Autodesk Inventor part; units mm, degrees
ref_plane "YZ Plane" through (0, 0, 0) normal (1, 0, 0) x (0, 1, 0)
ref_plane "XZ Plane" through (0, 0, 0) normal (0, 1, 0) x (-1, 0, 0)
ref_plane "XY Plane" through (0, 0, 0) normal (0, 0, 1) x (1, 0, 0)
sketch "Sketch1" plane through (0, 0, 0) normal (0, 1, 0) x (-1, 0, 0)
  line L0 (-24.384, 42.545) -> (24.384, 42.545)
  line L1 (24.384, 42.545) -> (24.384, -42.545)
  line L2 (24.384, -42.545) -> (-24.384, -42.545)
  line L3 (-24.384, -42.545) -> (-24.384, 42.545)
  line L4 (-24.384, 42.545) -> (24.384, -42.545) construction
  line L5 (24.384, 42.545) -> (-24.384, -42.545) construction
  line L6 (-12.7, 36.83) -> (12.7, 36.83)
  line L7 (12.7, 36.83) -> (12.7, -36.83)
  line L8 (12.7, -36.83) -> (-12.7, -36.83)
  line L9 (-12.7, -36.83) -> (-12.7, 36.83)
  line L10 (-12.7, 36.83) -> (12.7, -36.83) construction
  line L11 (12.7, 36.83) -> (-12.7, -36.83) construction
  line L12 (-24.384, 42.545) -> (-34.925, 42.545)
  line L13 (-34.925, 42.545) -> (-34.925, -42.545)
  line L14 (-34.925, -42.545) -> (-24.384, -42.545)
  line L15 (-24.384, -42.545) -> (-24.384, 42.545)
  circle A0 centre (15.494, 37.465) radius 1.5875
  circle A1 centre (-15.494, 37.465) radius 1.5875
  circle A2 centre (-15.494, -37.465) radius 1.5875
  circle A3 centre (15.494, -37.465) radius 1.5875
  point P0 (0, 0)
  dimension "d0" = 73.66
  dimension "d1" = 25.4
  dimension "d4" = 85.09
  dimension "d5" = 34.925
  dimension "d6" = 59.309
  dimension "d7" = 3.175
  dimension "d8" = 3.175
  dimension "d9" = 3.175
  dimension "d10" = 3.175
  dimension "d11" = 5.08
  dimension "d12" = 8.89
  dimension "d13" = 5.08
  dimension "d14" = 19.431
extrude "Extrusion1" add sketch "Sketch1" along normal blind 6.985
sketch "Sketch3" plane through (0, 0, 0) normal (0, -1, 0) x (1, 0, 0)
  line L0 (34.925, 42.545) -> (34.925, -42.545)
  line L1 (34.925, -42.545) -> (17.78, -42.545)
  line L2 (17.78, -42.545) -> (17.78, -5.715)
  line L3 (17.78, -5.715) -> (34.925, -5.715)
  line L4 (34.925, -5.715) -> (34.925, -42.545)
  point P0 (0, 0)
  point P1 (34.925, -5.715)
  dimension "d31" = 36.83
  dimension "d32" = 17.145
extrude "Extrusion3" add sketch "Sketch3" along normal blind 8.89
sketch "Sketch2" plane through (0, 6.985, 0) normal (0, 1, 0) x (1, 0, 0)
  circle A0 centre (21.59, 29.21) radius 3.0162
  circle A1 centre (28.194, 29.21) radius 3.0162
  circle A2 centre (24.638, 38.1) radius 3.0162
  circle A3 centre (24.638, 19.812) radius 3.0162
  line L0 (34.925, -42.545) -> (34.925, 42.545)
  circle A4 centre (24.638, 9.8298) radius 3.0162
  line L1 (34.925, 42.545) -> (-24.384, 42.545)
  point P0 (0, 0)
  dimension "d17" = 6.0325
  dimension "d18" = 6.0325
  dimension "d19" = 6.0325
  dimension "d20" = 6.0325
  dimension "d21" = 6.731
  dimension "d22" = 10.287
  dimension "d23" = 13.335
  dimension "d24" = 6.0325
  dimension "d25" = 4.445
  dimension "d26" = 18.288
  dimension "d27" = 8.89
  dimension "d28" = 28.2702
extrude "Extrusion2" cut sketch "Sketch2" against normal through all
sketch "Sketch7" plane through (-24.384, 0, -42.545) normal (0, 0, -1) x (-1, 0, 0)
  line L0 (-59.309, 6.985) -> (0, 6.985)
  line L1 (0, 0) -> (-59.309, 0)
  line L2 (0, 6.985) -> (-59.309, 6.985)
  line L3 (-59.309, 6.985) -> (-59.309, 0)
  line L4 (-59.309, 0) -> (0, 0)
  line L5 (0, 0) -> (0, 6.985)
  line L6 (-42.164, -8.89) -> (-59.309, -8.89)
  line L7 (-59.309, -8.89) -> (-42.164, -8.89)
  line L8 (-42.164, -8.89) -> (-42.164, 0)
  line L9 (-42.164, 0) -> (-59.309, 0)
  line L10 (-59.309, 0) -> (-59.309, -8.89)
  point P0 (-24.384, 0)
  point P1 (-45.4299, 3.81)
  point P2 (-45.4299, 3.81)
extrude "Extrusion5" add sketch "Sketch7" along normal blind 2.54
sketch "Sketch4" plane through (0, 6.985, 0) normal (0, 1, 0) x (1, 0, 0)
  circle A0 centre (21.59, 29.21) radius 3.0162
  circle A1 centre (21.59, 29.21) radius 5.715
  circle A2 centre (24.638, 38.1) radius 3.0162
  circle A3 centre (24.638, 38.1) radius 5.715
  circle A4 centre (28.194, 29.21) radius 3.0162
  circle A5 centre (24.638, 19.812) radius 3.0162
  circle A6 centre (24.638, 19.812) radius 5.715
  circle A7 centre (24.638, 9.8298) radius 3.0162
  circle A8 centre (24.638, 9.8298) radius 5.715
  circle A9 centre (28.194, 29.21) radius 5.715
  point P0 (0, 0)
  point P1 (24.892, 24.5455)
  point P2 (24.892, 33.8745)
  point P3 (23.8684, 25.4749)
  point P4 (23.108, 26.6036)
  point P5 (23.108, 31.8164)
  point P6 (23.518, 32.4958)
  point P7 (20.037, 34.71)
  point P8 (20.3805, 23.6245)
  point P9 (28.9636, 23.5471)
  point P10 (29.314, 34.8142)
  point P11 (26.191, 32.6)
  point P12 (26.676, 31.8164)
  point P13 (26.676, 26.6036)
  point P14 (25.8475, 25.3975)
  point P15 (21.8541, 14.8209)
  point P16 (27.4219, 14.8209)
  dimension "d35" = 11.43
  dimension "d36" = 11.43
  dimension "d37" = 11.43
  dimension "d38" = 11.43
  dimension "d39" = 11.43
fillet "Fillet1" radius 3.175 7 edges at (-24.384, 3.4925, 42.545) (34.925, 3.4925, 42.545) (34.925, -0.9525, -45.085) (-24.384, 3.4925, -45.085) (17.78, -4.445, -45.085) (17.78, -4.445, -5.715) (34.925, -4.445, -5.715)
equation "\"d8\" = d7"
equation "\"d9\" = d7"
equation "\"d10\" = d7"
equation "\"d18\" = d17"
equation "\"d19\" = d17"
equation "\"d20\" = d17"
equation "\"d24\" = d17"
equation "\"d36\" = d35"
equation "\"d37\" = d35"
equation "\"d38\" = d35"
equation "\"d39\" = d35"
properties part number "Button_Plate"
Model file for the job. Use its own axes, mm. A direction names the side the tool comes from. Coordinates: 2 decimals unless noted, no trailing zeros. Loops run counter-clockwise (first coordinate to the right, second up) from the corner with the lowest first, then second, coordinate; pieces in that order, holes last. Notation, with made-up numbers: (1, 63.5) -> (39, 63.5) arc R24 cw to (39, 98.5) -> close; hole circle Ø7 at (23, -20). An arc over 180 degrees is marked (long way). Answer as a JSON object with one key per item and string values.
Q1. Probe probe 1 along Z at (x, y) = (7.5, 2.75) (3 decimals); probe 2 along X at (y, z) = (1, -29.21) (3 decimals); probe 3 along Z at (x, y) = (23, -0.75) (3 decimals). List the from-to ranges inside material, lowest first.
Report:
{"probe 1": "z = -45.085 to -36.83, 36.83 to 42.545", "probe 2": "x = -24.384 to -12.7, 12.7 to 18.574, 24.606 to 25.178, 31.21 to 34.925", "probe 3": "z = -45.085 to -40.633, -35.567 to -31.876, -26.544 to -22.345, -17.279 to -12.362, -7.297 to -5.715"}
Q2. Cut at C-C (z = -29.21). List the corners of the cut face in (x, y) (3 decimals), and give its area (3 significant figures).
Report:
{"outline": "(-24.384, 0) -> (-12.7, 0) -> (-12.7, 6.985) -> (-24.384, 6.985) -> close; (12.7, 0) -> (17.78, 0) -> (17.78, -8.89) -> (18.574, -8.89) -> (18.574, 6.985) -> (12.7, 6.985) -> close; (24.606, -8.89) -> (25.178, -8.89) -> (25.178, 6.985) -> (24.606, 6.985) -> close; (31.21, -8.89) -> (34.925, -8.89) -> (34.925, 6.985) -> (31.21, 6.985) -> close", "area": "198 mm2"}
Q3. Cut at A-A (z = -1). List the corners of the cut face in (x, y) (3 decimals), and give its area (3 significant figures).
Report:
{"outline": "(-24.384, 0) -> (-12.7, 0) -> (-12.7, 6.985) -> (-24.384, 6.985) -> close; (12.7, 0) -> (34.925, 0) -> (34.925, 6.985) -> (12.7, 6.985) -> close", "area": "237 mm2"}
Q4. Cut at B-B (x = 2). List the corners of the cut face in (y, z) (3 decimals).
Report:
{"outline": "(0, -45.085) -> (6.985, -45.085) -> (6.985, -36.83) -> (0, -36.83) -> close; (0, 36.83) -> (6.985, 36.83) -> (6.985, 42.545) -> (0, 42.545) -> close"}
Q5. Pull direction Z, two halves, no side cores. Call faces 4 (the flat face through (17.78, -4, -26)), 5 (the cylindrical face through (18.735, -4.507, -6.62)), 6 (the cylindrical face through (14, 3, 38)): released by +Z, released by -Z, zero draft, split by the parting line, or undercut.
Report:
{"face 4": "zero draft", "face 5": "released by +Z", "face 6": "undercut"}
Q6. Cut at D-D (x = -15). List the corners of the cut face in (y, z) (3 decimals), and give its area (3 significant figures).
Report:
{"outline": "(0, -45.085) -> (6.985, -45.085) -> (6.985, -38.974) -> (0, -38.974) -> close; (0, -35.956) -> (6.985, -35.956) -> (6.985, 35.956) -> (0, 35.956) -> close; (0, 38.974) -> (6.985, 38.974) -> (6.985, 42.545) -> (0, 42.545) -> close", "area": "570 mm2"}
Q7. Flat gauge pins, fed straight in: P1, Ø9.5, axis at x = 24.64, z = -9.83, coming from the +Y side (3 decimals); P2, Ø3.5, axis at x = -15.494, z = -37.465, coming from the -Y side; P3, Ø4.5, axis at x = 25, y = -3, coming from the +Z side (3 decimals). Where does each tip first touch, or does it go through?
Report:
{"P1": "stops at y = 6.985", "P2": "stops at y = 0", "P3": "stops at z = -5.715"}
Q8. 3-axis set-ups, long thin cutter, end or side, ignore diameter. For faces 1 (the flat face through (26, -4, -5.715)), 2 (the cylindrical face through (18.735, -4.383, -44.18)), 3 (the flat face through (0, 3, 36.83)): which of +Z, -Z, +X, -X, +Y, -Y reach the whole face in a straight line?
Report:
{"face 1": "+Z, +X, -X, -Y", "face 2": "-Z, -X, -Y", "face 3": "+Y, -Y"}
